Autodesk Inventor part; units mm, degrees
ref_plane "YZ Plane" through (0, 0, 0) normal (1, 0, 0) x (0, 1, 0)
ref_plane "XZ Plane" through (0, 0, 0) normal (0, 1, 0) x (-1, 0, 0)
ref_plane "XY Plane" through (0, 0, 0) normal (0, 0, 1) x (1, 0, 0)
sketch "Эскиз1" plane through (0, 0, 0) normal (0, 1, 0) x (-1, 0, 0)
  circle A0 centre (0, 0) radius 7.45
  circle A1 centre (0, 0) radius 8.45
  line L0 (0, 0) -> (6.7429, 5.0927)
  line L1 (0, 0) -> (6.7429, -5.0927)
  point P0 (5.9449, -4.49)
  point P1 (5.9449, 4.49)
  dimension "d0" = 14.9
  dimension "d1" = 16.9
extrude "Выдавливание1" add sketch "Эскиз1" along normal blind 30 contours A0 L1 A1 L0 picked at (-7.9526, 1.3085)
sketch "Эскиз2" plane through (0, 30, 0) normal (0, 1, 0) x (1, 0, 0)
  arc A0 (-5.9449, -4.49) -> (-6.8376, -3.9601) centre (-8.6463, -8.0239) ccw
  arc A1 (-6.8376, -3.9601) -> (-7.9946, -5.7659) centre (-7.272, -4.9553) ccw
  line L0 (-7.9946, -5.7659) -> (-7.3233, -4.9114)
  arc A2 (-6.7444, -5.0781) -> (-7.3233, -4.9114) centre (-7.1127, -5.2686) ccw
  line L1 (-5.9449, -4.49) -> (-6.7429, -5.0927)
  line L2 (-6.7429, -5.0927) -> (-5.9449, -4.49)
  line L3 (-6.7429, -5.0927) -> (-6.7444, -5.0781)
  line L4 (-0.0151, 0) -> (-3.489, 0)
  arc A3 (-6.8376, 3.9601) -> (-5.9449, 4.49) centre (-8.6463, 8.0239) ccw
  arc A4 (-7.3233, 4.9114) -> (-6.7444, 5.0781) centre (-7.1127, 5.2686) ccw
  line L5 (-5.9449, 4.49) -> (-6.7429, 5.0927)
  line L6 (-6.7429, 5.0927) -> (-5.9449, 4.49)
  line L7 (-6.7429, 5.0927) -> (-6.7444, 5.0781)
  arc A5 (-7.9946, 5.7659) -> (-6.8376, 3.9601) centre (-7.272, 4.9553) ccw
  line L8 (-7.9946, 5.7659) -> (-7.3233, 4.9114)
  point P0 (-5.9449, 4.49)
  point P1 (-6.7429, -5.0927)
  point P2 (-5.3694, -4.0591)
  point P3 (-6.7429, 5.0927)
  point P4 (-5.3694, 4.0591)
  point P5 (-6.7429, 5.0927)
  dimension "d25" = 1.0859
sketch "Эскиз3" plane through (0, 30, 0) normal (0, 1, 0) x (1, 0, 0)
  arc A0 (-6.7429, -5.0927) -> (-6.7429, 5.0927) centre (0, 0) ccw
  line L0 (11.5, -6.95) -> (11.5, 6.95)
  arc A1 (-5.9449, -4.49) -> (-5.9449, 4.49) centre (0, 0) ccw
  line L1 (0, -8.45) -> (0, -7.45)
  line L2 (0, 7.45) -> (0, 8.45)
  line L3 (11.5, 6.95) -> (11.5, 10.95)
  line L4 (11.5, -6.95) -> (11.5, -10.95)
  line L5 (0, 3.95) -> (0, 8.45)
  line L6 (11.5, -10.95) -> (0, -10.95)
  line L7 (0, -10.95) -> (0, -8.45)
  line L8 (11.5, 10.95) -> (0, 10.95)
  line L9 (0, 10.95) -> (0, 8.45)
  arc A2 (0, -7.45) -> (0, 7.45) centre (0, 0) ccw
  dimension "d13" = 4
  dimension "d14" = 4
  dimension "d22" = 21.9
  dimension "d23" = 3.5
extrude "Выдавливание3" add sketch "Эскиз3" against normal blind 30
ref_plane "РабПлоскость1" through (11.5, 20, 4.95) normal (1, 0, 0) x (0, 0, -1)
sketch "Эскиз4" plane through (11.5, 20, 4.95) normal (1, 0, 0) x (0, 0, -1)
  line L0 (4.95, -20) -> (4.95, 10)
  line L1 (1, 10) -> (8.9, 10)
  circle A0 centre (4.95, -12) radius 5
  line L2 (14.4, -20) -> (-4.5, -20)
  circle A1 centre (4.95, 2) radius 5
  line L3 (-4.5, 10) -> (14.4, 10)
  point P0 (7.3306, 10)
  point P1 (2.5694, 10)
  point P2 (4.95, 10)
  dimension "d15" = 10
  dimension "d16" = 8
  dimension "d17" = 10
  dimension "d18" = 8
extrude "Выдавливание4" cut sketch "Эскиз4" against normal blind 2
extrude "Выдавливание5" add sketch "Эскиз2" against normal blind 30
sketch "Эскиз5" plane through (0, 30, 0) normal (0, 1, 0) x (1, 0, 0)
  arc A0 (0, 8.45) -> (-6.7429, 5.0927) centre (0, 0) ccw
  line L0 (-6.7429, 5.0927) -> (-6.7444, 5.0781)
  arc A1 (-7.3233, 4.9114) -> (-6.7444, 5.0781) centre (-7.1127, 5.2686) ccw
  line L1 (-7.3233, 4.9114) -> (-7.9946, 5.7659)
  arc A2 (-7.9946, 5.7659) -> (-6.8376, 3.9601) centre (-7.272, 4.9553) ccw
  arc A3 (-6.8376, 3.9601) -> (-5.9449, 4.49) centre (-8.6463, 8.0239) ccw
  arc A4 (-5.9449, -4.49) -> (-5.9449, 4.49) centre (0, 0) ccw
  arc A5 (-5.9449, -4.49) -> (-6.8376, -3.9601) centre (-8.6463, -8.0239) ccw
  arc A6 (-6.8376, -3.9601) -> (-7.9946, -5.7659) centre (-7.272, -4.9553) ccw
  line L2 (-7.9946, -5.7659) -> (-7.3233, -4.9114)
  arc A7 (-6.7444, -5.0781) -> (-7.3233, -4.9114) centre (-7.1127, -5.2686) ccw
  line L3 (-6.7444, -5.0781) -> (-6.7429, -5.0927)
  arc A8 (-6.7429, -5.0927) -> (0, -8.45) centre (0, 0) ccw
  line L4 (0, -8.45) -> (0, -10.95)
  line L5 (0, -10.95) -> (11.5, -10.95)
  line L6 (11.5, -10.95) -> (11.5, 10.95)
  line L7 (11.5, 10.95) -> (0, 10.95)
  line L8 (0, 10.95) -> (0, 8.45)
  line L9 (0, 7.45) -> (0, 8.45)
  line L10 (0, -7.45) -> (0, -8.45)
extrude "Выдавливание6" [suppressed]
sketch "Эскиз6" plane through (11.5, 30, 10.95) normal (1, 0, 0) x (0, 0, -1)
  arc A0 (15.95, -22) -> (15.95, -22) centre (10.95, -22) ccw
  arc A1 (15.95, -8) -> (15.95, -8) centre (10.95, -8) ccw
  point P0 (10.95, -30)
extrude "Выдавливание7" [suppressed]
properties part number "крепление маркера 15мм"
Input: part model. Units: mm. Frame: model coordinates. A direction names the side the tool comes from. Give positions to 0.01 mm unless a question says otherwise; leave off trailing zeros. Order: outer loops, then holes, each group sorted by start corner. A loop starts at its lowest first (then second) coordinate and runs counter-clockwise, first axis right, second up.
1. Draft query along Y for faces 5 (the face through (-7.66, 15.21, -5.34)), 6 (the face through (8, 30, 0)), 7 (the face through (9.5, 22, 0)). Return one class per face: released by +Y, released by -Y, zero draft, split by the parting line, or undercut.
Computed:
face 5: zero draft
face 6: released by +Y
face 7: undercut
2. Pin query (flat end, axial travel): pin 1 Ø1.5 at (y, z) = (16.5, 8) entering from -X; pin 2 Ø0.8 at (y, z) = (12.5, 10) entering from -X; pin 3 Ø1.5 at (x, y) = (-4.5, 13.5) entering from +Z. Return the tip coordinate at first contact, or that it passes through.
Computed:
pin 1: stops at x = -4.34
pin 2: stops at x = 0
pin 3: stops at z = 7.57
3. Cut plane D-D (z = 9). Return loops of the section in (x, y), and give its area (3 significant figures).
Computed:
outline: (0, 0) - (11.5, 0) - (11.5, 30) - (0, 30) - close
area: 345 mm2
4. Set-up query: faces 1 (the face through (0, 15, -10)), 2 (the face through (-6.382, 15.21, -4.195)), 3 (the face through (8, 0, 0)), 4 (the face through (9.5, 8, 0)). Return all of +Z, -Z, +X, -X, +Y, -Y with unobstructed straight access to the full face (end or side cutting, diameter ignored); none if empty.
Computed:
face 1: -Z, -X, +Y, -Y
face 2: +Y, -Y
face 3: +Z, -Z, +X, -X, -Y
face 4: +X
5. Line query: probe 1 along Y at (x, z) = (10.2, 0); probe 2 along Z at (x, y) = (10.85, 8); probe 3 along Y at (x, z) = (10.5, 2). Output: solid intervals per line, ascending.
Computed:
probe 1: y = 0 to 3, 13 to 17, 27 to 30
probe 2: z = -10.95 to -5, 5 to 10.95
probe 3: y = 0 to 3.42, 12.58 to 17.42, 26.58 to 30
6. Cut plane B-B (z = 0). Return loops of the section in (x, y), and give its area (3 significant figures).
Computed:
outline: (7.45, 0) - (11.5, 0) - (11.5, 3) - (9.5, 3) - (9.5, 13) - (11.5, 13) - (11.5, 17) - (9.5, 17) - (9.5, 27) - (11.5, 27) - (11.5, 30) - (7.45, 30) - close
area: 81.5 mm2
